Can you work these out from the model? Positions are in its coordinate system, mm. A direction names the side the tool comes from. Coordinates: 2 decimals unless noted, no trailing zeros. Loops run counter-clockwise (first coordinate to the right, second up) from the corner with the lowest first, then second, coordinate; pieces in that order, holes last. Notation, with made-up numbers: (20.25, 71.25) -> (61.25, 71.25) arc R19 ccw to (61.25, 81.25) -> close; hole circle Ø10 at (81.25, 2). An arc over 180 degrees is marked (long way). Put each result on its own line as item: value. Start each with the question number.
Item 1: We'd pull the mould along Z, two halves only. Please class faces 5 (the cylindrical face through (25.989, -0.285, 7.635)), 6 (the cylindrical face through (2.85, -9.62, 3.01)), 7 (the flat face through (53.22, -9.46, 87.82)): pulls with the +Z half, pulls with the -Z half, needs draft (parallel to the pull), parting line crosses it, or undercut.
Item 2: For faces 1 (the cylindrical face through (29.318, -18.715, 71.501)), 2 (the cylindrical face through (32.413, -2.105, 10.978)), 3 (the flat face through (31.493, -9.381, 72.409)), 4 (the flat face through (27.93, -9.38, 10)), which set-ups out of +Z, -Z, +X, -X, +Y, -Y let a thin tool reach every point of the face, with its end or its side?
Item 3: Please list where these lines run through material, in increasing order: L1, parallel to Y at x = 0.8, z = 30; L2, parallel to Z at x = 8, y = -6.75; L3, parallel to Z at x = 10.5, y = -1.5. Write a range as from..to.
Item 4: If we section it at A-A on z = 30: Please give me the cut outline in (x, y).
Item 5: Will these pins go through, and if not, where does the flat tip stop? P1, Ø4, axis at y = -8.5, z = 74.5, coming from the +X side; P2, Ø5, axis at y = -6, z = 39.5, coming from the +X side; P3, Ø5, axis at x = 6.5, y = -9.5, coming from the +Z side.
```python
from build123d import *

# Parameters (mm, degrees)
F1_DEPTH        = 19
F2_R            = 10
F3_R            = 5
F4_R            = 10
F5_R            = 10.1
F6_R            = 5
F7_R            = 10
F8_R            = 7
F9_R            = 7
F10_R           = 7
F11_R           = 1
F12_R           = 1
F14_D           = 4
F14_CSINK_D     = 7
F14_CSINK_ANGLE = 90


with BuildPart() as f1:
    # F0 (on Front) → F1 (new body)
    with BuildSketch(Plane.XZ):
        Polygon((0, 60), (0, 0), (25, 0), (35.606602, 10.606602), (32.071068, 14.142136), (22.928932, 5), (5, 5), (5, 57.113249), (54.461524, 85.669873), (51.961524, 90), align=None)
    extrude(amount=F1_DEPTH)

    # F2
    f2_edges = [f1.edges().sort_by_distance(p)[0] for p in [
        (5, -9.5, 57.113249),
    ]]
    fillet(f2_edges, radius=F2_R)

    # F3
    f3_edges = [f1.edges().sort_by_distance(p)[0] for p in [
        (5, -9.5, 5),
    ]]
    fillet(f3_edges, radius=F3_R)

    # F4
    f4_edges = [f1.edges().sort_by_distance(p)[0] for p in [
        (0, -9.5, 0),
    ]]
    fillet(f4_edges, radius=F4_R)

    # F5
    f5_edges = [f1.edges().sort_by_distance(p)[0] for p in [
        (0, -9.5, 60),
    ]]
    fillet(f5_edges, radius=F5_R)

    # F6
    f6_edges = [f1.edges().sort_by_distance(p)[0] for p in [
        (22.928932, -9.5, 5),
    ]]
    fillet(f6_edges, radius=F6_R)

    # F7
    f7_edges = [f1.edges().sort_by_distance(p)[0] for p in [
        (25, -9.5, 0),
    ]]
    fillet(f7_edges, radius=F7_R)

    # F8
    f8_edges = [f1.edges().sort_by_distance(p)[0] for p in [
        (53.211524, -19, 87.834936),
        (53.211524, 0, 87.834936),
    ]]
    fillet(f8_edges, radius=F8_R)

    # F9
    f9_edges = [f1.edges().sort_by_distance(p)[0] for p in [
        (33.838835, -19, 12.374369),
    ]]
    fillet(f9_edges, radius=F9_R)

    # F10
    f10_edges = [f1.edges().sort_by_distance(p)[0] for p in [
        (33.838835, 0, 12.374369),
    ]]
    fillet(f10_edges, radius=F10_R)

    # F11
    f11_edges = [f1.edges().sort_by_distance(p)[0] for p in [
        (25.474673, 0, 74.707809),
        (50.185953, -2.050253, 88.974874),
        (5.05, -9.5, 62.915619),
        (51.961524, -9.5, 90),
        (25.474673, -19, 74.707809),
        (50.185953, -16.949747, 88.974874),
    ]]
    fillet(f11_edges, radius=F11_R)

    # F12
    f12_edges = [f1.edges().sort_by_distance(p)[0] for p in [
        (32.071068, -9.5, 14.142136),
        (30.62132, -2.050253, 12.692388),
        (30.62132, -16.949747, 12.692388),
        (25.757359, 0, 7.828427),
        (25.757359, -19, 7.828427),
        (24.393398, -9.5, 6.464466),
    ]]
    fillet(f12_edges, radius=F12_R)

    # F14 (through all)
    with Locations(Plane.YZ.offset(5)):
        with Locations((-6, 41.339746), (-13, 30)):
            CounterSinkHole(F14_D / 2, F14_CSINK_D / 2, counter_sink_angle=F14_CSINK_ANGLE)


solid = f1.part
```
Solutions:
1. face 5: undercut
1. face 6: pulls with the -Z half
1. face 7: pulls with the +Z half
2. face 1: +X, -Y
2. face 2: +X, +Y
2. face 3: +X, +Y, -Y
2. face 4: +Y, -Y
3. L1: -18.98..-15, -11..-0.02
3. L2: 0.2..5.42, 58.48..64.62
3. L3: 0..5, 60.29..66.06
4. outline: (0, -18) arc R1 ccw to (1, -19) -> (4, -19) arc R1 ccw to (5, -18) -> (5, -16.5) -> (3.5, -15) -> (0, -15) -> close; (0, -11) -> (3.5, -11) -> (5, -9.5) -> (5, -1) arc R1 ccw to (4, 0) -> (1, 0) arc R1 ccw to (0, -1) -> close
5. P1: x = 38.58
5. P2: x = 5
5. P3: z = 65.2
